Design review of the part shown in the three views and the two pictorial views. Dimensions are in mm from the part's minimum x, y and z. A direction names the side the tool comes from. Coordinates: 2 decimals unless noted, no trailing zeros. Loops run counter-clockwise (first coordinate to the right, second up) from the corner with the lowest first, then second, coordinate; pieces in that order, holes last. Notation, with made-up numbers: M 74.5,49.5 L 128.5,49.5 A33 cw 128.5,79.5 Z; hole C 49.25,88.5 d9. An arc over 180 degrees is marked long. Answer as a JSON object with one key per item and string values. Group by question number.
Item 1: Mouldability with a two-part tool opening along X and no side actions: class the marked faces 3, 4 and 5 as +X half, -X half, draft (parallel to the pull), parting line (faces both ways), or undercut.
Item 2: Add section A-A (x = 5.5). State the section outline as (y, z) points (3 decimals).
Item 3: Add section C-C (y = 3.5). State the section outline as (x, z) points (3 decimals), then the cut area to 3 significant figures.
Item 4: Add section D-D (y = 6). State the section outline as (x, z) points, then the cut area to 3 significant figures.
Item 5: Wall thickness on L1, parallel to Z at x = 5.5, y = 1.4 (3 decimals); L2, parallel to X at y = 8, z = 4.75; L3, parallel to Y at x = 47.5, z = 6.5: over which ranges is each line inside the solid? List them lowest first. Write a range as from..to.
Item 6: Insertion check: pin 1 (1.5 mm diameter, centred on x = 35.5, z = 7.5, fed in from +Y); pin 2 (1.5 mm diameter, centred on x = 8.5, y = 5.5, fed in from -Z); pin 3 (1 mm diameter, centred on y = 8.5, z = 7, fed in from +X). Each pin has a flat end and moves straight along its axis. Give the tip position at first contact, or say it passes through.
Item 7: Add section B-B (z = 4.5). State the section outline as (x, y) points (3 decimals), then the cut area to 3 significant figures.
Item 8: Tool access review of the marked faces 1 and 2: name each direction out of +Z, -Z, +X, -X, +Y, -Y from which nothing blocks a thin tool from reaching the whole face with its end or side.
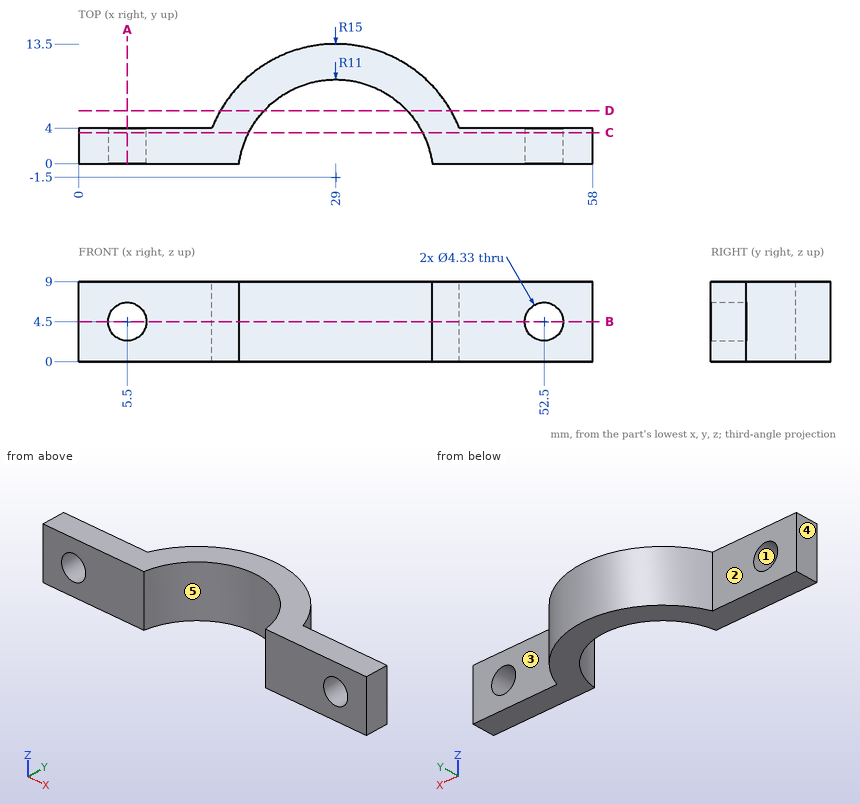
From the geometry:
{
 "1": {"face 3": "draft", "face 4": "-X half", "face 5": "undercut"},
 "2": {"outline": "M 0,0 L 4,0 L 4,2.335 L 0,2.335 Z; M 0,6.665 L 4,6.665 L 4,9 L 0,9 Z"},
 "3": {"outline": "M 0,0 L 19.202,0 L 19.202,9 L 0,9 Z; M 38.798,0 L 58,0 L 58,9 L 38.798,9 Z; hole C 5.5,4.5 d4.33; hole C 52.5,4.5 d4.33", "area": "316 mm²"},
 "4": {"outline": "M 16.01,0 L 20.95,0 L 20.95,9 L 16.01,9 Z; M 37.05,0 L 41.99,0 L 41.99,9 L 37.05,9 Z", "area": "89.0 mm²"},
 "5": {"L1": "z = 0..2.335, 6.665..9", "L2": "x = 17.39..23.45, 34.55..40.61", "L3": "y = 0..4"},
 "6": {"pin 1": "stops at y = 12.35", "pin 2": "passes through", "pin 3": "stops at x = 40.61"},
 "7": {"outline": "M 0,0 L 3.335,0 L 3.335,4 L 0,4 Z; M 7.665,0 L 18.103,0 A11 cw 39.897,0 L 50.335,0 L 50.335,4 L 42.955,4 A15 ccw 15.045,4 L 7.665,4 Z; M 54.665,0 L 58,0 L 58,4 L 54.665,4 Z", "area": "232 mm²"},
 "8": {"face 1": "+Y, -Y", "face 2": "+Z, -Z, -X, +Y"}
}
